Answer from the drawing. Dimensions are ordinates in mm from the lowest x, y and z of the part. Coordinates: 2 decimals unless noted, no trailing zeros. Loops run counter-clockwise (first coordinate to the right, second up) from the corner with the lowest first, then second, coordinate; pieces in that order, holes last. Notation, with made-up numbers: M -19.75,-17 L 23.25,-17 A34 cw 23.25,17 Z; hole C 13,72 d6. An arc over 180 degrees is marked long. Put each result on its own line as item: value.
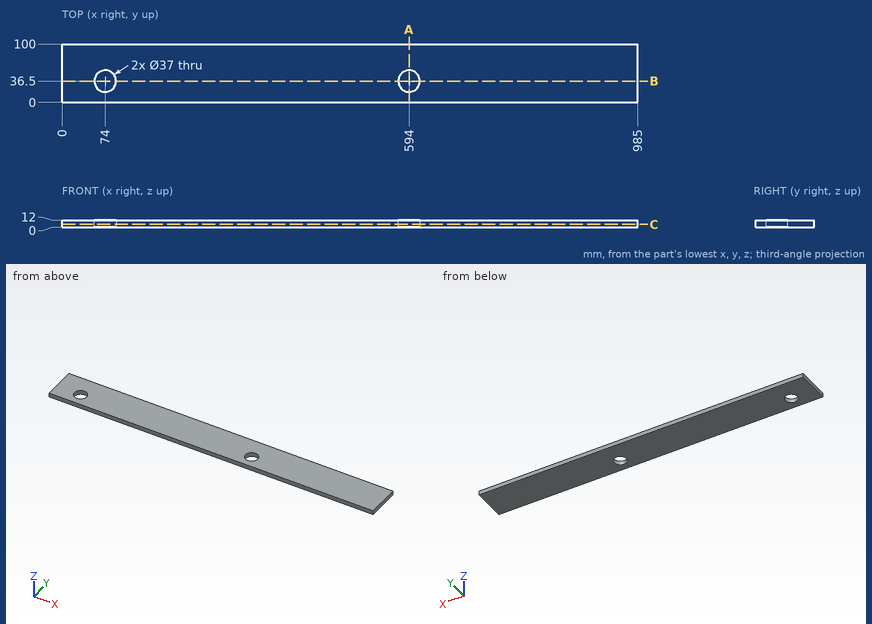
1) Find section B-B, the plane y = 36.5. Write down the section's boundary in (x, z), plus the area to 3 significant figures.
Answer list:
outline: M 0,0 L 55.5,0 L 55.5,12 L 0,12 Z; M 92.5,0 L 575.5,0 L 575.5,12 L 92.5,12 Z; M 612.5,0 L 985,0 L 985,12 L 612.5,12 Z
area: 10,900 mm^2
2) Straight lines are drawn through the part: line 1 (Y direction, x = 74, z = 5); line 2 (X direction, y = 20, z = 3.25); line 3 (X direction, y = 26, z = 5.25). For each, find the intervals that lie inside material, in ascending order. Write a range as [from, to].
Answer list:
line 1: y = [0, 18], [55, 100]
line 2: x = [0, 65.63], [82.37, 585.63], [602.37, 985]
line 3: x = [0, 58.77], [89.23, 578.77], [609.23, 985]
3) Find section C-C, the plane z = 5.25. Write down the section's boundary in (x, y), plus the area to 3 significant figures.
Answer list:
outline: M 0,0 L 985,0 L 985,100 L 0,100 Z; hole C 74,36.5 d37; hole C 594,36.5 d37
area: 96,300 mm^2
4) Find section A-A, the plane x = 594. Write down the section's boundary in (y, z).
Answer list:
outline: M 0,0 L 18,0 L 18,12 L 0,12 Z; M 55,0 L 100,0 L 100,12 L 55,12 Z
5) Given pin 1 Ø22 at (x, y) = (74, 36.5) entering from +Z, flat-ended and moving along its own axis, determine where the tip first touches the part or whether it passes through.
Answer list:
pin 1: passes through
